Autodesk Inventor part; units mm, degrees
ref_plane "YZ Plane" through (0, 0, 0) normal (1, 0, 0) x (0, 1, 0)
ref_plane "XZ Plane" through (0, 0, 0) normal (0, 1, 0) x (-1, 0, 0)
ref_plane "XY Plane" through (0, 0, 0) normal (0, 0, 1) x (1, 0, 0)
sketch "Sketch5" plane through (0, 0, 0) normal (0, 0, 1) x (1, 0, 0)
  circle A0 centre (0, 0) radius 3.175
  line L0 (0, 3.175) -> (7.9375, 3.175)
  line L1 (0, -3.175) -> (7.9375, -3.175)
  line L2 (7.9375, 3.175) -> (38.1, 0)
  line L3 (38.1, 0) -> (7.9375, -3.175)
  dimension "d16" = 6.35
  dimension "d17" = 7.9375
  dimension "d18" = 7.9375
  dimension "d19" = 38.1
extrude "Extrusion2" add sketch "Sketch5" along normal blind 28.575
sketch "Sketch6" plane through (0, 0, 0) normal (0, 0, -1) x (-1, 0, 0)
  circle A0 centre (0, 0) radius 1.5875
  dimension "d22" = 3.175
sketch "Sketch7" plane through (0, 0, 0) normal (0, 1, 0) x (-1, 0, 0)
  line L0 (0, 0) -> (0, 3.175)
  line L1 (-7.9375, 11.1125) -> (-9.4615, 11.1125)
  arc A0 (0, 3.175) -> (-7.9375, 11.1125) centre (-7.9375, 3.175) ccw
  dimension "d23" = 3.175
  dimension "d26" = 1.524
  dimension "d27" = 7.9375
  dimension "d28" = 7.9375
sweep "Sweep2" cut profiles "Sketch6" path "Sketch7"
fillet "Fillet1" radius 25.4 2 edges at (7.9375, 3.175, 14.2875) (7.9375, -3.175, 14.2875)
properties part number "foreDivePlanes" material "ABS Plastic"
Input: part model. Units: mm. Frame: model coordinates. A direction names the side the tool comes from. Coordinates: 2 decimals unless noted, no trailing zeros. Order: outer loops, then holes, each group sorted by start corner. A loop starts at its lowest first (then second) coordinate and runs counter-clockwise, first axis right, second up. Notation, with made-up numbers: M 24,-37.75 L 47,-37.75 A22 ccw 47,-1.75 Z; hole C 4,-1.75 d11. An arc over 180 degrees is marked long. Answer as CSV lines item,"result".
1. Material intervals for line 1 (Z direction, x = 8.9, y = 0) (3 decimals); line 2 (Y direction, x = -1, z = 1.5); line 3 (Y direction, x = 34, z = 22), sorted ascending. Write a range as from..to.
Reported:
line 1,"0..9.525, 12.7..28.575"
line 2,"-3.01..-1.23, 1.23..3.01"
line 3,"-0.43..0.43"
2. Section A-A (z = 24.5). Return the cut outline in (x, y) (3 decimals).
Reported:
outline,"M 0,-3.175 L 6.604,-3.175 A25.4 ccw 9.263,-3.035 L 38.1,0 L 9.263,3.035 A25.4 ccw 6.604,3.175 L 0,3.175 A3.175 ccw Z"
3. Pull-direction query (Y, two-part tool) for faces 4 (the flat face through (23.884, -1.496, 14.087)), 5 (the flat face through (13, 0, 28.575)), 6 (the cylindrical face through (8.71, -0.477, 12.627)); classes: released by +Y, released by -Y, zero draft, split by the parting line, or undercut.
Reported:
face 4,"released by -Y"
face 5,"zero draft"
face 6,"undercut"
4. Section B-B (x = 20.5). Return the cut outline in (y, z) (3 decimals).
Reported:
outline,"M -1.853,0 L 1.853,0 L 1.853,28.575 L -1.853,28.575 Z"
5. Access query for faces 1 (the flat face through (9.462, 0, 11)), 2 (the flat face through (23.48, 1.54, 14.09)), 3 (the cylindrical face through (0.34, 1.55, 1.61)). Directions: +Z, -Z, +X, -X, +Y, -Y. A direction counts if a zero-diameter tool reaches every point of the face in a straight line with its end or side. Return the directions, or none.
Reported:
face 1,"none"
face 2,"+Z, -Z, +X, +Y"
face 3,"-Z"
6. First-contact query: P1, Ø5, axis at x = 9.5, z = 6, coming from the -Y side; P2, Ø2, axis at x = 32.5, z = 4.5, coming from the -Y side. Flat tips, straight axial feed; report the tip coordinate or a pass-through.
Reported:
P1,"y = -3.17"
P2,"y = -0.69"
